CAD build for the part. Positions are in the model's coordinates, mm. Face numbers are marked on the shaded views. A direction names the side the tool comes from. Give positions to 0.01 mm unless a question says otherwise; leave off trailing zeros. Write each loop counter-clockwise with the first axis right and the second up, starting at its lowest first coordinate (ties: lowest second). Pieces come first, ordered by that corner, then holes. Notation, with made-up numbers: (37, -25) -> (89, -25) arc R24 cw to (89, -6) -> close; hole circle Ø1 at (-0.5, 61). An arc over 180 degrees is marked (long way). Answer in a Markdown table with one row per item. Add a question column.
```python
from build123d import *

# Parameters (mm, degrees)
SKETCH1_R           = 40.656565244
BOSS_EXTRUDE2_DEPTH = 143
BOSS_EXTRUDE2_TAPER = 3
SKETCH2_R           = 49
BOSS_EXTRUDE3_DEPTH = 20
FILLET1_R           = 5
BOSS_EXTRUDE4_START = 143
BOSS_EXTRUDE4_DEPTH = 12
BOSS_EXTRUDE5_START = 155
SKETCH4_R           = 6
BOSS_EXTRUDE5_DEPTH = 18
BOSS_EXTRUDE5_TAPER = 3


with BuildPart() as part:
    # Sketch1 → Boss-Extrude2 (new body)
    with BuildSketch(Plane(origin=(0, 0, 0), x_dir=(1, 0, 0), z_dir=(0, 1, 0))):
        Circle(SKETCH1_R)
    extrude(amount=BOSS_EXTRUDE2_DEPTH, taper=BOSS_EXTRUDE2_TAPER)

    # Sketch2 → Boss-Extrude3 (add)
    with BuildSketch(Plane(origin=(0, 0, 0), x_dir=(-1, 0, 0), z_dir=(0, -1, 0))):
        Circle(SKETCH2_R)
    extrude(amount=BOSS_EXTRUDE3_DEPTH)

    # Fillet1
    fillet1_edges = [part.edges().sort_by_distance(p)[0] for p in [
        (49, -20, 0),
    ]]
    fillet(fillet1_edges, radius=FILLET1_R)

    # Sketch3 → Boss-Extrude4 (add)
    with BuildSketch(Plane(origin=(0, 0, 0), x_dir=(1, 0, 0), z_dir=(0, 1, 0)).offset(BOSS_EXTRUDE4_START)):
        Polygon((6.639528096, -11.5), (13.279056191, 0), (6.639528096, 11.5), (-6.639528096, 11.5), (-13.279056191, 0), (-6.639528096, -11.5), align=None)
    extrude(amount=BOSS_EXTRUDE4_DEPTH)

    # Sketch4 → Boss-Extrude5 (add)
    with BuildSketch(Plane(origin=(0, 0, 0), x_dir=(1, 0, 0), z_dir=(0, 1, 0)).offset(BOSS_EXTRUDE5_START)):
        Circle(SKETCH4_R)
    extrude(amount=BOSS_EXTRUDE5_DEPTH, taper=BOSS_EXTRUDE5_TAPER)


solid = part.part
```
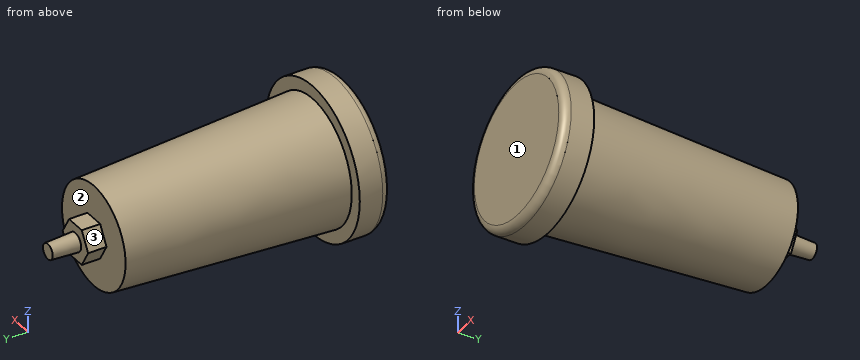
Item 1: Slice it at B-B, the plane y = 149.5. List the corners of the cut face in (x, z), then the cut area to 3 significant figures.
Item 2: Slice it at D-D, the plane y = 85. List the corners of the cut face in (x, z).
Item 3: Which spindle directions (+Z, -Z, +X, -X, +Y, -Y) get a long thin tool onto all of the face, cutting with end or side? Do the marked faces 1, 2 and 3. Say none if no direction does.
Item 4: Slice it at A-A, the plane x = 0. List the corners of the cut face in (y, z), then the cut area to 3 significant figures.
Item 5: Slice it at C-C, the plane y = 4.5. List the corners of the cut face in (x, z).
Item 6: Drop flat-ended pins along their axis: pin 1 Ø4 at (y, z) = (103.5, 23) entering from -X; pin 2 Ø4 at (y, z) = (107.5, -27.5) entering from -X; pin 3 Ø6 at (x, y) = (-0.5, 147.5) entering from -Z; pin 4 Ø18.5 at (x, z) = (-5.5, 0) entering from +Y. Give the stop position or say it passes through.
Item 7: Probe L1, parallel to Y at x = -22, z = -13.5; L2, parallel to X at y = 139, z = -30; L3, parallel to Z at x = 36, y = 19.5. List the from-to ranges inside material, lowest first. Write a range as from..to.
Answer key:
| question | item | result |
|---|---|---|
| 1 | outline | (-13.28, 0) -> (-6.64, -11.5) -> (6.64, -11.5) -> (13.28, 0) -> (6.64, 11.5) -> (-6.64, 11.5) -> close |
| 1 | area | 458 mm² |
| 2 | outline | circle Ø72.4 at (0, 0) |
| 3 | face 1 | +Z, -Z, +X, -X, -Y |
| 3 | face 2 | +Y |
| 3 | face 3 | +Z, -X, +Y |
| 4 | outline | (-20, -44) arc R5 ccw to (-15, -49) -> (0, -49) -> (0, -40.66) -> (143, -33.16) -> (143, -11.5) -> (155, -11.5) -> (155, -6) -> (173, -5.06) -> (173, 5.06) -> (155, 6) -> (155, 11.5) -> (143, 11.5) -> (143, 33.16) -> (0, 40.66) -> (0, 49) -> (-15, 49) arc R5 ccw to (-20, 44) -> close |
| 4 | area | 13,000 mm² |
| 5 | outline | circle Ø80.84 at (0, 0) |
| 6 | pin 1 | stops at x = -28.3 |
| 6 | pin 2 | stops at x = -24.01 |
| 6 | pin 3 | stops at z = -11.5 |
| 6 | pin 4 | stops at y = 173 |
| 7 | L1 | y = -20..143 |
| 7 | L2 | x = -14.62..14.62 |
| 7 | L3 | z = -16.58..16.58 |
